Input: dimensioned drawing with shaded views. Units: mm. Origin: part minimum x, y, z. A direction names the side the tool comes from. Coordinates: 2 decimals unless noted, no trailing zeros. Loops run counter-clockwise (first coordinate to the right, second up) from the corner with the lowest first, then second, coordinate; pieces in that order, holes last. Notation, with made-up numbers: (87, 4) -> (98, 4) arc R30 cw to (98, 41) -> close; hole circle Ø5 at (70, 19). An arc over 180 degrees is marked (long way). Answer as CSV lines item,"result".
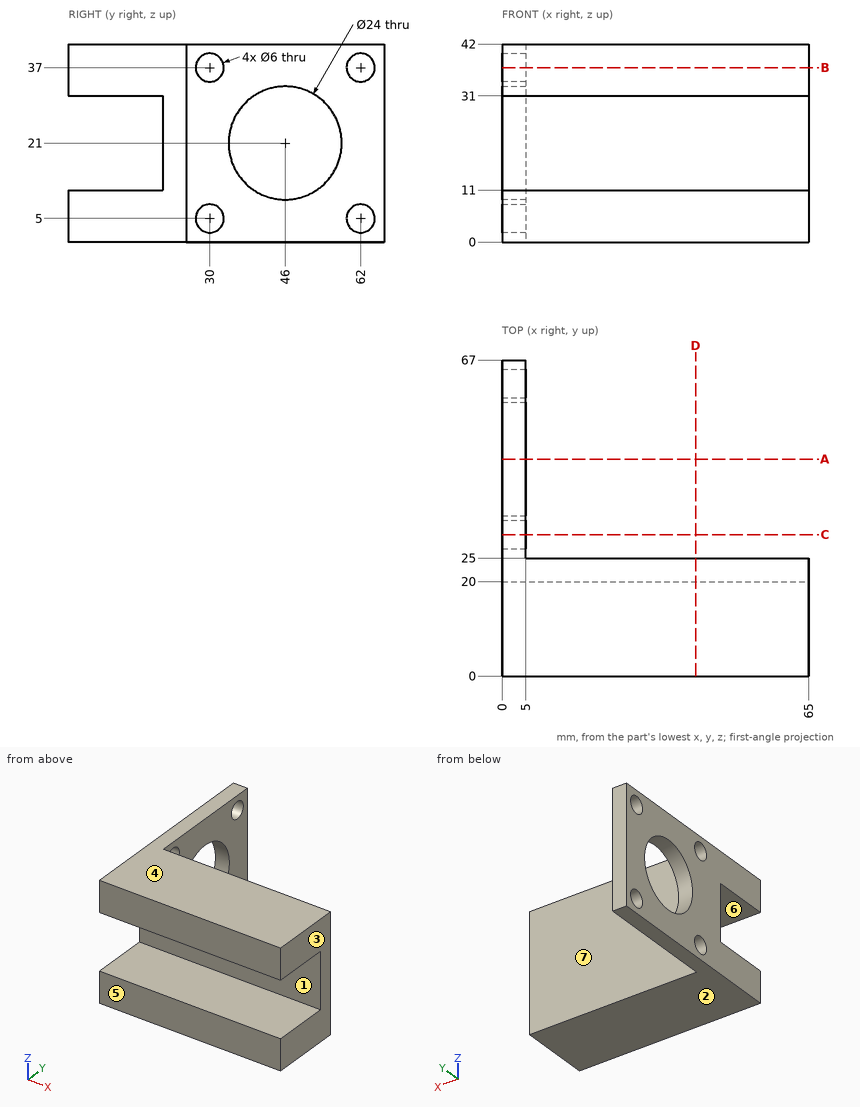
(1) Pin query (flat end, axial travel): pin 1 Ø21 at (x, z) = (36.5, 31) entering from +Y; pin 2 Ø22 at (x, y) = (34, 12.5) entering from -Z; pin 3 Ø9.5 at (y, z) = (62, 5) entering from +X; pin 4 Ø6 at (x, z) = (36.5, 16.5) entering from -Y. Return the tip coordinate at first contact, or that it passes through.
Computed values:
pin 1,"y = 25"
pin 2,"z = 0"
pin 3,"x = 5"
pin 4,"y = 20"
(2) Draft query along Z for the marked faces 1, 2, 3 and 4. Return one class per face: released by +Z, released by -Z, zero draft, split by the parting line, or undercut.
Computed values:
face 1,"undercut"
face 2,"released by -Z"
face 3,"zero draft"
face 4,"released by +Z"
(3) Cut plane B-B (z = 37). Return the cut outline in (x, y), then the cut area to 4 significant figures.
Computed values:
outline,"(0, 0) -> (65, 0) -> (65, 25) -> (5, 25) -> (5, 27) -> (0, 27) -> close; (0, 33) -> (5, 33) -> (5, 59) -> (0, 59) -> close; (0, 65) -> (5, 65) -> (5, 67) -> (0, 67) -> close"
area,"1,775 mm^2"
(4) Material intervals for L1, parallel to Y at x = 3, z = 5; L2, parallel to Z at x = 34.5, y = 14.5; L3, parallel to Y at x = 53, z = 25, sorted ascending. Write a range as [from, to].
Computed values:
L1,"[0, 27], [33, 59], [65, 67]"
L2,"[0, 11], [31, 42]"
L3,"[20, 25]"
(5) Cut plane C-C (y = 30). Return the cut outline in (x, z).
Computed values:
outline,"(0, 0) -> (5, 0) -> (5, 2) -> (0, 2) -> close; (0, 8) -> (5, 8) -> (5, 34) -> (0, 34) -> close; (0, 40) -> (5, 40) -> (5, 42) -> (0, 42) -> close"
(6) Cut plane D-D (x = 41). Return the cut outline in (y, z), then the cut area to 3 significant figures.
Computed values:
outline,"(0, 0) -> (25, 0) -> (25, 42) -> (0, 42) -> (0, 31) -> (20, 31) -> (20, 11) -> (0, 11) -> close"
area,"650 mm^2"
(7) Cut plane A-A (y = 46). Return the cut outline in (x, z), then the cut area to 3 significant figures.
Computed values:
outline,"(0, 0) -> (5, 0) -> (5, 9) -> (0, 9) -> close; (0, 33) -> (5, 33) -> (5, 42) -> (0, 42) -> close"
area,"90.0 mm^2"
(8) Access query for the marked faces 5, 6 and 7. Directions: +Z, -Z, +X, -X, +Y, -Y. A direction counts if a zero-diameter tool reaches every point of the face in a straight line with its end or side. Return the directions, or none.
Computed values:
face 5,"+Z, -Z, +X, -X, -Y"
face 6,"+X, -X, -Y"
face 7,"+Z, -Z, +X, +Y"
